Autodesk Inventor part; units mm, degrees
ref_plane "YZ Plane" through (0, 0, 0) normal (1, 0, 0) x (0, 1, 0)
ref_plane "XZ Plane" through (0, 0, 0) normal (0, 1, 0) x (-1, 0, 0)
ref_plane "XY Plane" through (0, 0, 0) normal (0, 0, 1) x (1, 0, 0)
sketch "Boceto1" plane through (0, 0, 0) normal (0, 1, 0) x (-1, 0, 0)
  line L0 (-11.7171, -8.4187) -> (-13.9671, -8.4187)
  line L1 (-13.9671, -8.4187) -> (-13.9671, -17.4187)
  line L2 (-13.9671, -17.4187) -> (-11.7171, -17.4187)
  line L3 (-11.7171, -17.4187) -> (-11.7171, -25.8375)
  line L4 (-11.7171, -25.8375) -> (-3.9546, -25.8375)
  line L5 (-3.9546, -25.8375) -> (-3.9546, -28.0875)
  line L6 (-3.9546, -28.0875) -> (5.0454, -28.0875)
  line L7 (5.0454, -28.0875) -> (5.0454, -25.8375)
  line L8 (5.0454, -25.8375) -> (11.6829, -25.8375)
  line L9 (11.6829, -25.8375) -> (11.6829, -17.4194)
  line L10 (11.6829, -17.4194) -> (13.9329, -17.4187)
  line L11 (13.9329, -17.4187) -> (13.9329, -8.4187)
  line L12 (13.9329, -8.4187) -> (11.6829, -8.4187)
  line L13 (11.6829, -8.4187) -> (11.6829, 8.4188)
  line L14 (11.6829, 8.4188) -> (13.9329, 8.4188)
  line L15 (13.9329, 8.4188) -> (13.9329, 17.4188)
  line L16 (13.9329, 17.4188) -> (11.6829, 17.4188)
  line L17 (11.6829, 17.4188) -> (11.6829, 21.3375)
  line L18 (11.6829, 21.3375) -> (11.6829, 25.8375)
  line L19 (11.6829, 25.8375) -> (5.0454, 25.8375)
  line L20 (5.0454, 25.8375) -> (5.0454, 28.0875)
  line L21 (5.0454, 28.0875) -> (-3.9546, 28.0875)
  line L22 (-3.9546, 28.0875) -> (-3.9546, 25.8375)
  line L23 (-3.9546, 25.8375) -> (-10.5921, 25.8375)
  line L24 (-10.5921, 25.8375) -> (-10.9671, 25.8375)
  line L25 (-10.9671, 25.8375) -> (-11.7171, 25.8375)
  line L26 (-11.7171, 25.8375) -> (-11.7171, 17.4188)
  line L27 (-11.7171, 17.4188) -> (-13.9671, 17.4188)
  line L28 (-13.9671, 17.4188) -> (-13.9671, 8.4188)
  line L29 (-13.9671, 8.4188) -> (-11.7171, 8.4188)
  line L30 (-11.7171, 8.4188) -> (-11.7171, -8.4187)
extrude "Extrusión1" add sketch "Boceto1" along normal blind 2.4
properties part number "costat2"
Read the model definition and answer for the solid it produces. Units are mm, in the model's axes. A direction names the side the tool comes from. Give positions to 0.01 mm unless a question says otherwise; leave off trailing zeros. Loops run counter-clockwise (first coordinate to the right, second up) from the corner with the lowest first, then second, coordinate; pieces in that order, holes last.
Item 1: The part is cut by section B-B (x = 10.5). Write down the section's boundary in (y, z), and give its area (3 significant figures).
Item 2: The part is cut by section C-C (z = -1.5). Write down the section's boundary in (x, y).
Item 3: The part is cut by section A-A (y = 1.1). Write down the section's boundary in (x, z), and give its area (3 significant figures).
Item 4: Each of these flat-tipped pins is pushed along its axis until it touches: pin 1 Ø1.1 at (x, y) = (-13, 1.5) entering from -Z; pin 2 Ø0.7 at (x, y) = (-13, 2) entering from +Z; pin 3 Ø1 at (x, y) = (10, 1) entering from +Z. Where does it stop, or does it pass through?
Item 5: The mould has two halves that part along Z. Classify faces 1 (the flat face through (-13, 1, -8.419)), 2 (the flat face through (13, 1, -17.419)), 3 (the flat face through (13.967, 1, 13)), 4 (the flat face through (-11.683, 1, 0)): released by +Z, released by -Z, zero draft, split by the parting line, or undercut.
Item 6: For faces 5 (the flat face through (11.717, 1, -22)), 6 (the flat face through (-13, 1, 17.419)), 7 (the flat face through (-5.045, 1, -27)), 8 (the flat face through (13, 1, -8.419)), 9 (the flat face through (11.717, 1, 22)), determine the directions among +Z, -Z, +X, -X, +Y, -Y from which every point of the face is accessible in a straight line to the end or side of a thin tool.
Item 7: Find the intervals of material crossed by line 1 along Z through (x, y) = (-11.75, 0.9); line 2 along Z through (x, y) = (-7.5, 2.05); line 3 along X through (y, z) = (0.2, 19), in increasing order.
Taken from the geometry:
1. outline: (0, -25.84) - (2.4, -25.84) - (2.4, 25.84) - (0, 25.84) - close
1. area: 124 mm2
2. outline: (-11.68, 0) - (11.72, 0) - (11.72, 2.4) - (-11.68, 2.4) - close
3. outline: (-13.93, -17.42) - (-11.68, -17.42) - (-11.68, -25.84) - (-5.05, -25.84) - (-5.05, -28.09) - (3.95, -28.09) - (3.95, -25.84) - (11.72, -25.84) - (11.72, -17.42) - (13.97, -17.42) - (13.97, -8.42) - (11.72, -8.42) - (11.72, 8.42) - (13.97, 8.42) - (13.97, 17.42) - (11.72, 17.42) - (11.72, 25.84) - (3.95, 25.84) - (3.95, 28.09) - (-5.05, 28.09) - (-5.05, 25.84) - (-11.68, 25.84) - (-11.68, 17.42) - (-13.93, 17.42) - (-13.93, 8.42) - (-11.68, 8.42) - (-11.68, -8.42) - (-13.93, -8.42) - close
3. area: 1,330 mm2
4. pin 1: stops at z = -17.42
4. pin 2: stops at z = 17.42
4. pin 3: stops at z = 25.84
5. face 1: undercut
5. face 2: released by -Z
5. face 3: zero draft
5. face 4: undercut
6. face 5: -Z, +X, +Y, -Y
6. face 6: +Z, -X, +Y, -Y
6. face 7: -Z, -X, +Y, -Y
6. face 8: +X, +Y, -Y
6. face 9: +Z, +X, +Y, -Y
7. line 1: z = -17.42 to -8.42, 8.42 to 17.42
7. line 2: z = -25.84 to 25.84
7. line 3: x = -11.68 to 11.72
